For this review, take the finished solid that the model builds, in its own axes (mm). Coordinates: 2 decimals unless noted, no trailing zeros. Loops run counter-clockwise (first coordinate to the right, second up) from the corner with the lowest first, then second, coordinate; pieces in that order, holes last. Notation, with made-up numbers: (-5, 83) - (29, 83) arc R24 ccw to (29, 96) - close; hole circle Ø7 at (79.25, 53). An arc over 180 degrees is marked (long way). Use one line per item in the form item = value. Start each with the question number.
1. Add section D-D on y = 9.5. Give the boundary of the cut face in (x, z), and give its area (3 significant figures).
2. Add section C-C on z = 0.1. Give the boundary of the cut face in (x, y), and give its area (3 significant figures).
3. Add section B-B on y = 58.5. Give the boundary of the cut face in (x, z).
4. Add section A-A on x = -63.5. Give the boundary of the cut face in (y, z).
5. To check wall thickness, follow probe 1 along X at (y, z) = (69.5, 0.15); probe 2 along Y at (x, z) = (-58, 0.15); probe 3 along X at (y, z) = (15.5, 0.1). State the ranges of each line that lie inside material, in increasing order.
```python
from build123d import *

# Parameters (mm, degrees)
PAD_DEPTH          = 0.2
POLARPATTERN_COUNT = 4


with BuildPart() as part:
    # Sketch → Pad (new body)
    with BuildSketch(Plane(origin=(0, 0, 0), x_dir=(0.707107, 0.707107, 0), z_dir=(0, 0, 1))):
        Polygon((0, 120), (10, 120), (10, 10), (120, 10), (120, 0), (0, 0), align=None)
    pad = extrude(amount=PAD_DEPTH)

    # PolarPattern: Pad ×4 about axis
    polarpattern_axis = Axis((0, 0, 0), (0, 0, 1))
    for i in range(1, POLARPATTERN_COUNT):
        add(pad.rotate(polarpattern_axis, i * 360 / POLARPATTERN_COUNT))


solid = part.part
```
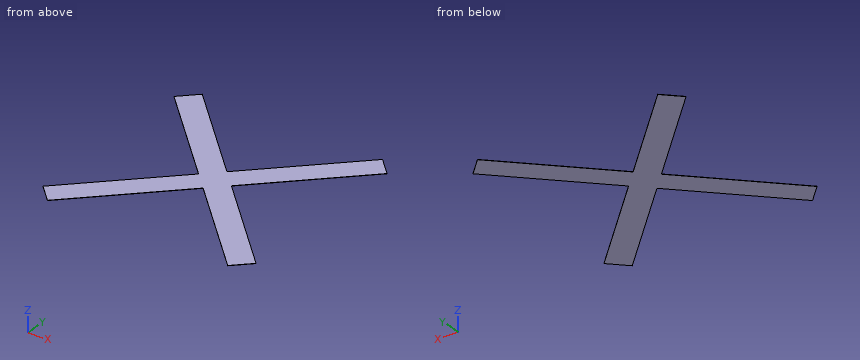
Conclusion:
q1.outline = (-23.64, 0) - (23.64, 0) - (23.64, 0.2) - (-23.64, 0.2) - close
q1.area = 9.46 mm^2
q2.outline = (-91.92, -77.78) - (-77.78, -91.92) - (0, -14.14) - (77.78, -91.92) - (91.92, -77.78) - (14.14, 0) - (91.92, 77.78) - (77.78, 91.92) - (0, 14.14) - (-77.78, 91.92) - (-91.92, 77.78) - (-14.14, 0) - close
q2.area = 9,200 mm^2
q3.outline = (-72.64, 0) - (-44.36, 0) - (-44.36, 0.2) - (-72.64, 0.2) - close; (44.36, 0) - (72.64, 0) - (72.64, 0.2) - (44.36, 0.2) - close
q4.outline = (-77.64, 0) - (-49.36, 0) - (-49.36, 0.2) - (-77.64, 0.2) - close; (49.36, 0) - (77.64, 0) - (77.64, 0.2) - (49.36, 0.2) - close
q5.probe_1 = -83.64 to -55.36, 55.36 to 83.64
q5.probe_2 = -72.14 to -43.86, 43.86 to 72.14
q5.probe_3 = -29.64 to -1.36, 1.36 to 29.64
